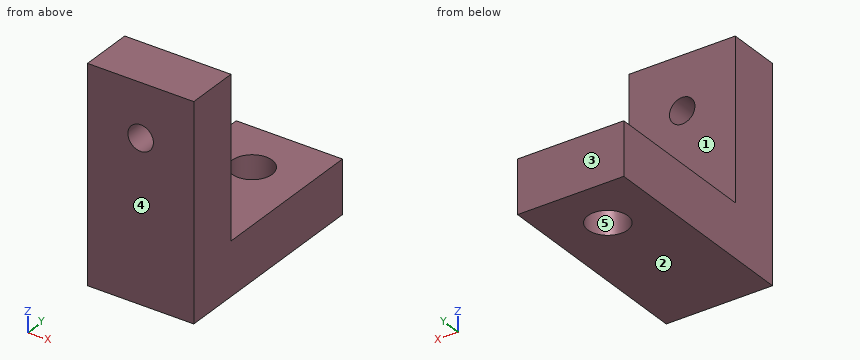
from build123d import *

# Parameters (mm, degrees)
SKETCH1_R           = 2.38125
BOSS_EXTRUDE1_DEPTH = 6.35
SKETCH2_W           = 12.7
SKETCH2_H           = 6.35
BOSS_EXTRUDE2_DEPTH = 19.05
SKETCH3_R           = 1.524
CUT_EXTRUDE1_DEPTH  = 19.05


with BuildPart() as part:
    # Sketch1 → Boss-Extrude1 (new body)
    with BuildSketch(Plane.XY):
        Polygon((-6.35, 0), (-6.35, -19.05), (6.35, -19.05), (6.35, 0), (6.35, 6.35), (-6.35, 6.35), align=None)
        Circle(SKETCH1_R, mode=Mode.SUBTRACT)
    extrude(amount=BOSS_EXTRUDE1_DEPTH)

    # Sketch2 → Boss-Extrude2 (add)
    with BuildSketch(Plane.XY.offset(6.35)):
        with Locations((0, -15.875)):
            Rectangle(SKETCH2_W, SKETCH2_H)
    extrude(amount=BOSS_EXTRUDE2_DEPTH)

    # Sketch3 → Cut-Extrude1 (cut)
    with BuildSketch(Plane(origin=(0, -12.7, 0), x_dir=(1, 0, 0), z_dir=(0, 1, 0))):
        with Locations(Location((0, -19.05, 0), (0, 0, 270))):
            Circle(SKETCH3_R)
    extrude(amount=-CUT_EXTRUDE1_DEPTH, mode=Mode.SUBTRACT)


solid = part.part
Here's how the part is built. I have some questions about the finished solid (model axes, mm). Face numbers are marked on the shaded views. A direction names the side the tool comes from. Round coordinates to 2 decimals unless told otherwise and drop trailing zeros. Order: outer loops, then holes, each group sorted by start corner. A loop starts at its lowest first (then second) coordinate and runs counter-clockwise, first axis right, second up. Notation, with made-up numbers: (-27.5, 81.25) -> (6.5, 81.25) arc R8 cw to (6.5, 95.25) -> close; hole circle Ø9 at (-14.5, -22.75). An arc over 180 degrees is marked (long way). Return JSON: item names as keys, results as strings.
Q1. If we section it at D-D on z = 4.25: List the corners of the cut face in (x, y) for me, plus the area to 3 significant figures.
Filled sheet:
{"outline": "(-6.35, -19.05) -> (6.35, -19.05) -> (6.35, 6.35) -> (-6.35, 6.35) -> close; hole circle Ø4.76 at (0, 0)", "area": "305 mm^2"}
Q2. If we section it at C-C on y = 0: List the corners of the cut face in (x, z) for me, plus the area to 3 significant figures.
Filled sheet:
{"outline": "(-6.35, 0) -> (-2.38, 0) -> (-2.38, 6.35) -> (-6.35, 6.35) -> close; (2.38, 0) -> (6.35, 0) -> (6.35, 6.35) -> (2.38, 6.35) -> close", "area": "50.4 mm^2"}
Q3. If we section it at B-B on z = 19.05: List the corners of the cut face in (x, y) for me.
Filled sheet:
{"outline": "(-6.35, -19.05) -> (-1.52, -19.05) -> (-1.52, -12.7) -> (-6.35, -12.7) -> close; (1.52, -19.05) -> (6.35, -19.05) -> (6.35, -12.7) -> (1.52, -12.7) -> close"}
Q4. If we section it at A-A on x = 0: List the corners of the cut face in (y, z) for me, plus the area to 3 significant figures.
Filled sheet:
{"outline": "(-19.05, 0) -> (-2.38, 0) -> (-2.38, 6.35) -> (-12.7, 6.35) -> (-12.7, 17.53) -> (-19.05, 17.53) -> close; (-19.05, 20.57) -> (-12.7, 20.57) -> (-12.7, 25.4) -> (-19.05, 25.4) -> close; (2.38, 0) -> (6.35, 0) -> (6.35, 6.35) -> (2.38, 6.35) -> close", "area": "233 mm^2"}
Q5. For pin 1 Ø6.5 at (x, y) = (-2.5, -6) entering from +Z; pin 2 Ø1 at (x, z) = (5, 16) entering from +Y, each with a flat end and sliding along its axis, tell me the tip position at first contact or that it passes through.
Filled sheet:
{"pin 1": "stops at z = 6.35", "pin 2": "stops at y = -12.7"}
Q6. I need wall thicknesses on line 1 along X through (y, z) = (-17.5, 19.05); line 2 along Y through (x, z) = (-2.75, 12); line 3 along Z through (x, y) = (-4.5, -6.75). Which ranges of each line are inside material? Lowest first, please. Write a range as from..to.
Filled sheet:
{"line 1": "x = -6.35..-1.52, 1.52..6.35", "line 2": "y = -19.05..-12.7", "line 3": "z = 0..6.35"}
Q7. If we mould it in two halves opening along Y, with no side actions, what happens to the marked faces 3, 4 and 5? For each: released by +Y, released by -Y, zero draft, split by the parting line, or undercut.
Filled sheet:
{"face 3": "released by +Y", "face 4": "released by -Y", "face 5": "undercut"}
Q8. Which directions (+Z, -Z, +X, -X, +Y, -Y) give clear straight access to the entire face, cutting with the end or side of a thin tool? Please do the marked faces 1 and 2.
Filled sheet:
{"face 1": "+Z, +X, -X, +Y", "face 2": "-Z, +X, -X, +Y, -Y"}
